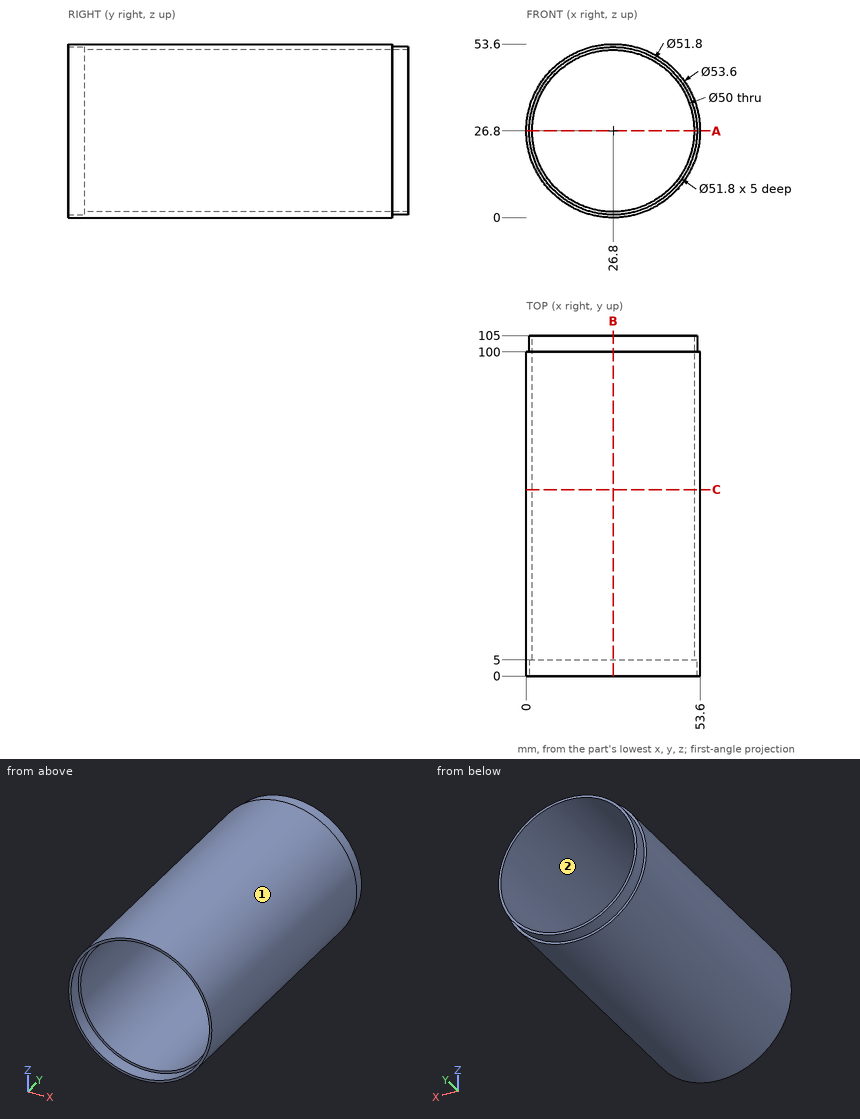
Here's the drawing with two shaded views (mm, measured from the low corner). I have some questions. Coordinates: 2 decimals unless noted, no trailing zeros. Loops run counter-clockwise (first coordinate to the right, second up) from the corner with the lowest first, then second, coordinate; pieces in that order, holes last. Notation, with made-up numbers: M 55.25,73 L 82.25,73 A38 cw 82.25,112 Z; hole C -12.5,5 d3. An arc over 180 degrees is marked long. Put each result on its own line as item: value. Start each with the question number.
(1) Imagine slicing it at A-A on z = 26.8. List the corners of the cut face in (x, y) for me.
(2) Imagine slicing it at C-C on y = 57.5. List the corners of the cut face in (x, z) for me.
(3) Will these pins go through, and if not, where does the flat tip stop? pin 1 Ø2 at (y, z) = (93, 43.5) entering from +X; pin 2 Ø8 at (x, y) = (15.5, 72) entering from -Z; pin 3 Ø1.5 at (x, y) = (47, 38.5) entering from -Z.
(4) We'd pull the mould along Z, two halves only. Please class the marked faces 1 and 2: +Z half, -Z half, draft (parallel to the pull), parting line (faces both ways), or undercut.
(5) I need wall thicknesses on probe 1 along Z at (x, y) = (26, 29); probe 2 along Z at (x, y) = (26, 1); probe 3 along X at (y, z) = (91.5, 8.5). Which ranges of each line are inside material? Lowest first, please.
(6) Imagine slicing it at B-B on x = 26.8. List the corners of the cut face in (y, z) for me, and give its area (3 significant figures).
Worked answers:
1. outline: M 0,0 L 0.9,0 L 0.9,5 L 1.8,5 L 1.8,105 L 0.9,105 L 0.9,100 L 0,100 Z; M 51.8,5 L 52.7,5 L 52.7,0 L 53.6,0 L 53.6,100 L 52.7,100 L 52.7,105 L 51.8,105 Z
2. outline: C 26.8,26.8 d53.6; hole C 26.8,26.8 d50
3. pin 1: stops at x = 48.52
3. pin 2: stops at z = 1.01
3. pin 3: stops at z = 8.36
4. face 1: parting line
4. face 2: undercut
5. probe 1: z = 0.01 to 1.81, 51.79 to 53.59
5. probe 2: z = 0.01 to 0.91, 52.69 to 53.59
5. probe 3: x = 7.22 to 9.77, 43.83 to 46.38
6. outline: M 0,0 L 100,0 L 100,0.9 L 105,0.9 L 105,1.8 L 5,1.8 L 5,0.9 L 0,0.9 Z; M 0,52.7 L 5,52.7 L 5,51.8 L 105,51.8 L 105,52.7 L 100,52.7 L 100,53.6 L 0,53.6 Z
6. area: 360 mm2
